Part print with two shaded views. Sizes in mm from the minimum x, y, z corner. A direction names the side the tool comes from. Round coordinates to 2 decimals unless told otherwise and drop trailing zeros. Order: outer loops, then holes, each group sorted by start corner. A loop starts at its lowest first (then second) coordinate and runs counter-clockwise, first axis right, second up. Notation, with made-up numbers: M -30,-40 L 26,-40 A27 cw 26,-7 Z; hole C 42.5,8.5 d6. An arc over 180 degrees is marked long. Put each result on its own line as item: value.
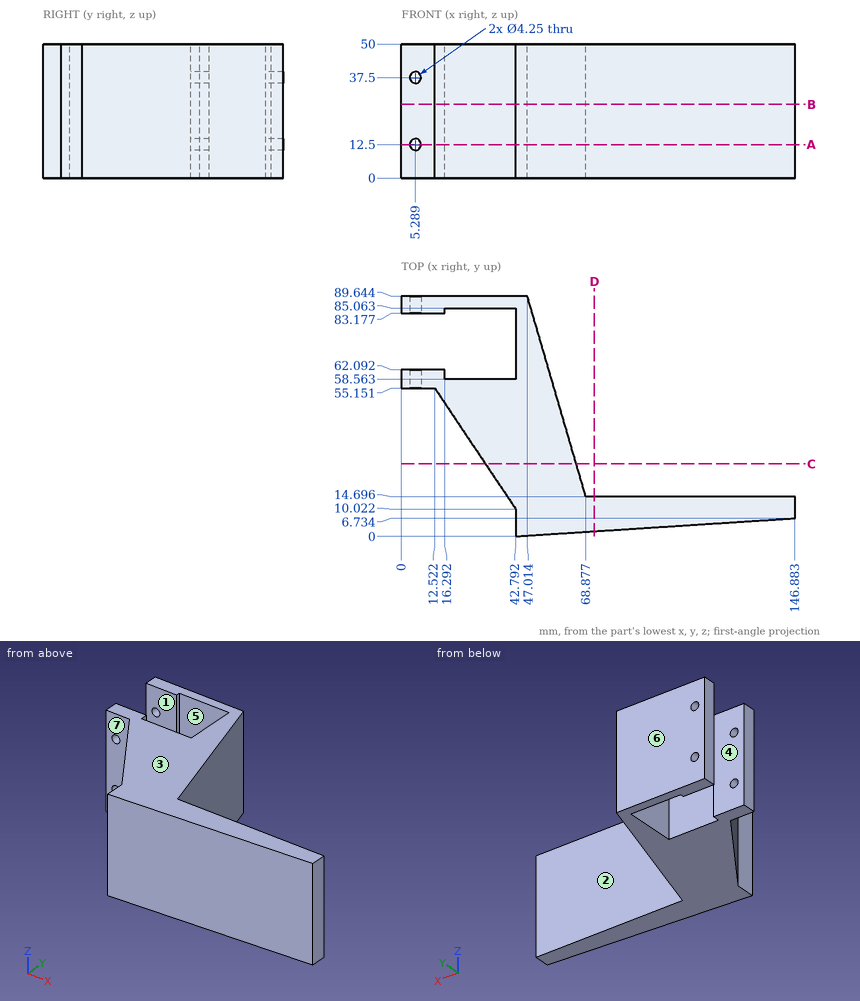
Item 1: Probe line 1 along X through (y, z) = (59, 12) (1 decimal); line 2 along Y through (x, z) = (26, 18.5) (1 decimal); line 3 along Y through (x, z) = (28.5, 27.5) (1 decimal). List the from-to ranges inside material, lowest first. Write a range as [from, to].
Answers below:
line 1: [0, 3.2], [7.4, 16.3], [42.8, 56]
line 2: [35.1, 58.6], [85.1, 89.6]
line 3: [31.3, 58.6], [85.1, 89.6]
Item 2: Mould opens along Y. For the marked faces 1, 2 and 3 say: pulls with the +Y half, pulls with the -Y half, needs draft (parallel to the pull), parting line crosses it, or undercut.
Answers below:
face 1: undercut
face 2: pulls with the +Y half
face 3: needs draft
Item 3: Band-saw the part on C-C on y = 27. Give the cut face in (x, z) (1 decimal).
Answers below:
outline: M 31.4,0 L 65.3,0 L 65.3,50 L 31.4,50 Z
Item 4: Pin check, flat tips, straight feed: P1, Ø3, axis at y = 4.5, z = 24.5, coming from the -X side; P2, Ø25, axis at x = 96.5, z = 25, coming from the +Y side; P3, Ø1.5, axis at y = 84.5, z = 21.5, coming from the +X side. Stop position of each tip, or through.
Answers below:
P1: x = 42.79
P2: y = 14.7
P3: x = 48.73
Item 5: Tool access for the marked faces 4, 5, 6 and 7: list every direction of +Z, -Z, +X, -X, +Y, -Y with a clear straight run to the whole face (end or side of a thin tool).
Answers below:
face 4: +Z, -Z, -X
face 5: +Z, -Z
face 6: +Z, -Z, +X, -X, +Y
face 7: +Z, -Z, -X, -Y
Item 6: Band-saw the part on D-D on x = 72. Give the cut face in (y, z), and give its area (3 significant figures).
Answers below:
outline: M 1.89,0 L 14.7,0 L 14.7,50 L 1.89,50 Z
area: 640 mm²
Item 7: Band-saw the part on B-B on z = 27.5. Give the cut face in (x, y) (1 decimal), and give its area (3 significant figures).
Answers below:
outline: M 0,55.2 L 12.5,55.2 L 42.8,10 L 42.8,0 L 146.9,6.7 L 146.9,14.7 L 68.9,14.7 L 47,89.6 L 0,89.6 L 0,83.2 L 16.3,83.2 L 16.3,85.1 L 42.8,85.1 L 42.8,58.6 L 16.3,58.6 L 16.3,62.1 L 0,62.1 Z
area: 3,430 mm²
Item 8: Band-saw the part on A-A on z = 12.5. Give the cut face in (x, y) (1 decimal), and give its area (3 significant figures).
Answers below:
outline: M 0,55.2 L 3.2,55.2 L 3.2,62.1 L 0,62.1 Z; M 0,83.2 L 3.2,83.2 L 3.2,89.6 L 0,89.6 Z; M 7.4,55.2 L 12.5,55.2 L 42.8,10 L 42.8,0 L 146.9,6.7 L 146.9,14.7 L 68.9,14.7 L 47,89.6 L 7.4,89.6 L 7.4,83.2 L 16.3,83.2 L 16.3,85.1 L 42.8,85.1 L 42.8,58.6 L 16.3,58.6 L 16.3,62.1 L 7.4,62.1 Z
area: 3,370 mm²
